Design review of the part built by this model. Coordinates are the model's own, in mm. A direction names the side the tool comes from. Round coordinates to 2 decimals unless told otherwise and drop trailing zeros. Loops run counter-clockwise (first coordinate to the right, second up) from the corner with the lowest first, then second, coordinate; pieces in that order, holes last. Notation, with made-up numbers: M 40,38.5 L 63,38.5 A23 cw 63,57.5 Z; hole C 21,52 d1. An arc over 180 degrees is marked long. Use a Markdown table: item, result.
from build123d import *

# Parameters (mm, degrees)
F0_W        = 100
F0_H        = 70
F0_R        = 22.5
F1_DEPTH    = 25
F2_R        = 4.25
F3_DEPTH    = 25.001
F4_SIZE     = 2.5
F5_T1_DEPTH = 77.8584149398
F5_T3_DEPTH = 30.6428543011
F5_T5_DEPTH = 107.8584149398
F6_W        = 0.4621222615
F6_H        = 1.904300414
F7_DEPTH    = 25


# Not quite as in the source:
# - a fillet or chamfer that OpenCascade refuses, or shapes differently, is made with other operations: its cross-section is extruded or revolved along the edge and cut away or added


with BuildPart() as f1:
    # F0 (on Top) → F1 (new body)
    with BuildSketch(Plane.XY):
        Rectangle(F0_W, F0_H)
        Circle(F0_R, mode=Mode.SUBTRACT)
    extrude(amount=F1_DEPTH)

    # F2 (on face) → F3 (cut, through all)
    with BuildSketch(Plane.XY.offset(25)):
        with Locations((-40, 25)):
            Circle(F2_R)
        with Locations((-40, -25)):
            Circle(F2_R)
        with Locations((40, -25)):
            Circle(F2_R)
        with Locations((40, 25)):
            Circle(F2_R)
    extrude(amount=-F3_DEPTH, mode=Mode.SUBTRACT)

    # F4
    f4_edges = [f1.edges().sort_by_distance(p)[0] for p in [
        (50, 35, 12.5),
        (50, -35, 12.5),
        (-50, -35, 12.5),
        (-50, 35, 12.5),
    ]]
    chamfer(f4_edges, length=F4_SIZE)

    # F5: chamfer of 2.5 on 16 edges, made by hand

    # F5_s2 → F5_t1 (cut)
    with BuildSketch(Plane.XZ.offset(-38.9292074699)):
        Polygon((47.5, 25), (50, 22.5), (50, 25), align=None)
        Polygon((47.5, 0), (50, 2.5), (50, 0), align=None)
        Polygon((-47.5, 0), (-50, 2.5), (-50, 0), align=None)
        Polygon((-47.5, 25), (-50, 22.5), (-50, 25), align=None)
    extrude(amount=F5_T1_DEPTH, mode=Mode.SUBTRACT)

    # F5_s4 → F5_t3 (cut)
    with BuildSketch(Plane.XY.offset(-2.8214271505)):
        Polygon((49.267766953, -33.232233047), (50, -31.4644660941), (50, -32.5), align=None)
        Polygon((50, 31.4644660941), (49.267766953, 33.232233047), (50, 32.5), align=None)
        Polygon((-46.4644660941, -35), (-48.232233047, -34.267766953), (-47.5, -35), align=None)
        Polygon((46.4644660941, -35), (48.232233047, -34.267766953), (47.5, -35), align=None)
        Polygon((-50, 31.4644660941), (-49.267766953, 33.232233047), (-50, 32.5), align=None)
        Polygon((-49.267766953, -33.232233047), (-50, -31.4644660941), (-50, -32.5), align=None)
        Polygon((48.232233047, 34.267766953), (46.4644660941, 35), (47.5, 35), align=None)
        Polygon((-48.232233047, 34.267766953), (-46.4644660941, 35), (-47.5, 35), align=None)
    extrude(amount=F5_T3_DEPTH, mode=Mode.SUBTRACT)

    # F5_s6 → F5_t5 (cut)
    with BuildSketch(Plane.YZ.offset(-53.9292074699)):
        Polygon((-35, 2.5), (-32.5, 0), (-35, 0), align=None)
        Polygon((-35, 22.5), (-32.5, 25), (-35, 25), align=None)
        Polygon((32.5, 0), (35, 2.5), (35, 0), align=None)
        Polygon((32.5, 25), (35, 22.5), (35, 25), align=None)
    extrude(amount=F5_T5_DEPTH, mode=Mode.SUBTRACT)

    # F6 (on face) → F7 (join)
    with BuildSketch(Plane.XY.offset(25)):
        Polygon((-33.0991968513, 1.4772834256), (-33.0991968513, -8.5106156766), (-27.7881808579, -8.5106156766), (-27.7881808579, 11.4651825279), (-33.0991968513, 11.4651825279), (-33.0991968513, 3.3815838397), (-32.6370745897, 3.3815838397), (-32.6370745897, 1.4772834256), align=None)
        with Locations((-32.8681357205, 2.4294336326)):
            Rectangle(F6_W, F6_H)
    extrude(amount=F7_DEPTH)


solid = f1.part
1. Take a section at B-B on x = 40. Give the boundary of the cut face in (y, z), and give its area (3 significant figures).
Check values:
| item | result |
|---|---|
| outline | M -35,2.5 L -32.5,0 L -29.25,0 L -29.25,25 L -32.5,25 L -35,22.5 Z; M -20.75,0 L 20.75,0 L 20.75,25 L -20.75,25 Z; M 29.25,0 L 32.5,0 L 35,2.5 L 35,22.5 L 32.5,25 L 29.25,25 Z |
| area | 1,310 mm² |
2. Take a section at C-C on x = 0. Give the boundary of the cut face in (y, z).
Check values:
| item | result |
|---|---|
| outline | M -35,2.5 L -32.5,0 L -22.5,0 L -22.5,25 L -32.5,25 L -35,22.5 Z; M 22.5,0 L 32.5,0 L 35,2.5 L 35,22.5 L 32.5,25 L 22.5,25 Z |
3. Wall thickness on line 1 along Y through (x, z) = (-40, 9.25); line 2 along Y through (x, z) = (41, 7); line 3 along Z through (x, y) = (-10.5, -30): over which ranges is each line inside the solid? List them lowest first. Write a range as from..to.
Check values:
| item | result |
|---|---|
| line 1 | y = -35..-29.25, -20.75..20.75, 29.25..35 |
| line 2 | y = -35..-29.13, -20.87..20.87, 29.13..35 |
| line 3 | z = 0..25 |
4. Insertion check: pin 1 (7.5 mm diameter, centred on x = -40, y = -25, fed in from +Z); pin 2 (6 mm diameter, centred on x = -9.5, y = 25, fed in from +Z); pin 3 (6 mm diameter, centred on x = -30.5, z = 43.5, fed in from +Y); pin 4 (16 mm diameter, centred on y = -1, z = 43, fed in from +X). Each pin has a flat end and moves straight along its axis. Give the tip position at first contact, or say it passes through.
Check values:
| item | result |
|---|---|
| pin 1 | passes through |
| pin 2 | stops at z = 25 |
| pin 3 | stops at y = 11.47 |
| pin 4 | stops at x = -27.79 |
5. Machinability: for faces 5 (the face through (-30, -8.511, 37)), 6 (the face through (-22, 8, 0)), which of the approach directions +Z, -Z, +X, -X, +Y, -Y give a long, thin tool a straight path to every point of the face, cutting with its end or side? Answer none if there is none.
Check values:
| item | result |
|---|---|
| face 5 | +Z, +X, -X, -Y |
| face 6 | -Z, +X, -X, +Y, -Y |
6. Take a section at A-A on y = -25. Give the boundary of the cut face in (x, z), and give its area (3 significant figures).
Check values:
| item | result |
|---|---|
| outline | M -50,2.5 L -47.5,0 L -44.25,0 L -44.25,25 L -47.5,25 L -50,22.5 Z; M -35.75,0 L 35.75,0 L 35.75,25 L -35.75,25 Z; M 44.25,0 L 47.5,0 L 50,2.5 L 50,22.5 L 47.5,25 L 44.25,25 Z |
| area | 2,060 mm² |
7. Take a section at D-D on z = 8. Give the boundary of the cut face in (x, y), and give its area (3 significant figures).
Check values:
| item | result |
|---|---|
| outline | M -50,-31.46 L -49.27,-33.23 L -48.23,-34.27 L -46.46,-35 L 46.46,-35 L 48.23,-34.27 L 49.27,-33.23 L 50,-31.46 L 50,31.46 L 49.27,33.23 L 48.23,34.27 L 46.46,35 L -46.46,35 L -48.23,34.27 L -49.27,33.23 L -50,31.46 Z; hole C -40,-25 d8.5; hole C -40,25 d8.5; hole C 0,0 d45; hole C 40,-25 d8.5; hole C 40,25 d8.5 |
| area | 5,170 mm² |
8. The part is to be moulded in two halves that separate along Y. For faces 1 (the face through (-44.246, -24.813, 12.675)), 2 (the face through (-30, 11.465, 37)), 3 (the face through (-0.7, -33.8, 1.3)), 4 (the face through (-33.099, 2, 37)), say which applies: pulls with the +Y half, pulls with the -Y half, needs draft (parallel to the pull), parting line crosses it, or undercut.
Check values:
| item | result |
|---|---|
| face 1 | undercut |
| face 2 | pulls with the +Y half |
| face 3 | pulls with the -Y half |
| face 4 | needs draft |
